Answer from the drawing. Dimensions are ordinates in mm from the lowest x, y and z of the part. A direction names the side the tool comes from. Coordinates: 2 decimals unless noted, no trailing zeros. Loops run counter-clockwise (first coordinate to the right, second up) from the corner with the lowest first, then second, coordinate; pieces in that order, holes last. Notation, with made-up numbers: M 13,19 L 56,19 A18 ccw 56,33 Z; hole C 70,57 d7. An arc over 180 degrees is marked long. Put each result on its own line as item: value.
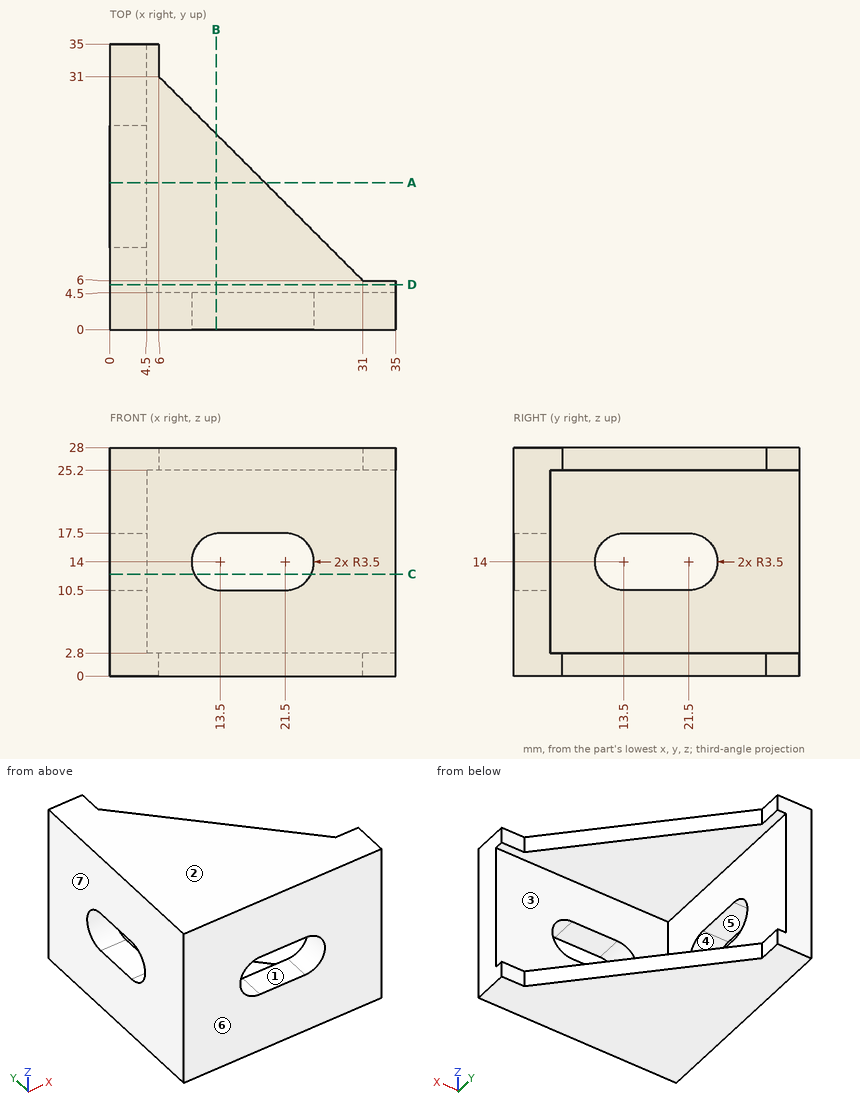
1) Given pin 1 Ø3 at (x, z) = (33.5, 27) entering from +Y; pin 2 Ø11 at (x, z) = (16, 16.5) entering from +Y; pin 3 Ø3 at (y, z) = (32, 2) entering from +X, each flat-ended and moving along its own axis, determine where each tip first touches the part or whether it passes through.
Answer list:
pin 1: stops at y = 6
pin 2: stops at y = 4.5
pin 3: stops at x = 6.5
2) Find section A-A, the plane y = 18. Write down the section's boundary in (x, z).
Answer list:
outline: M 0,0 L 19,0 L 19,2.8 L 4.5,2.8 L 4.5,10.5 L 0,10.5 Z; M 0,17.5 L 4.5,17.5 L 4.5,25.2 L 19,25.2 L 19,28 L 0,28 Z
3) Determine the mould class of the marked faces 5, 6 and 7 for opening direction Y: released by +Y, released by -Y, zero draft, split by the parting line, or undercut.
Answer list:
face 5: undercut
face 6: released by -Y
face 7: zero draft
4) Straight lines are drawn through the part: line 1 (Z direction, x = 11, y = 10); line 2 (Z direction, x = 16, y = 1); line 3 (X direction, y = 9, z = 5.5). For each, find the intervals that lie inside material, in ascending order. Write a range as [from, to].
Answer list:
line 1: z = [0, 2.8], [25.2, 28]
line 2: z = [0, 10.5], [17.5, 28]
line 3: x = [0, 4.5]
5) Which of the six approach directions +Z, -Z, +X, -X, +Y, -Y give full straight-line access (tool end or side, diameter ignored) to the marked faces 1, 2, 3 and 4?
Answer list:
face 1: +Y, -Y
face 2: +Z, +X, -X, +Y, -Y
face 3: +X, +Y
face 4: +X, -X
6) Find section C-C, the plane z = 12.5. Write down the section's boundary in (x, y).
Answer list:
outline: M 0,0 L 10.34,0 L 10.34,4.5 L 4.5,4.5 L 4.5,10.34 L 0,10.34 Z; M 0,24.66 L 4.5,24.66 L 4.5,35 L 0,35 Z; M 24.66,0 L 35,0 L 35,4.5 L 24.66,4.5 Z
7) Find section B-B, the plane x = 13. Write down the section's boundary in (y, z), plus the area to 3 significant figures.
Answer list:
outline: M 0,0 L 24,0 L 24,2.8 L 4.5,2.8 L 4.5,10.54 L 0,10.54 Z; M 0,17.46 L 4.5,17.46 L 4.5,25.2 L 24,25.2 L 24,28 L 0,28 Z
area: 204 mm^2
8) Find section D-D, the plane y = 5.5. Write down the section's boundary in (x, z), plus the area to 3 significant figures.
Answer list:
outline: M 0,0 L 35,0 L 35,2.8 L 4.5,2.8 L 4.5,25.2 L 35,25.2 L 35,28 L 0,28 Z
area: 297 mm^2
